The drawing under review shows one solid part. Ordinate dimensions are in mm from its lowest x, y, z. A direction names the side the tool comes from. Coordinates: 2 decimals unless noted, no trailing zeros. Write each loop counter-clockwise with the first axis right and the second up, starting at its lowest first coordinate (ties: lowest second). Pieces come first, ordered by that corner, then holes.
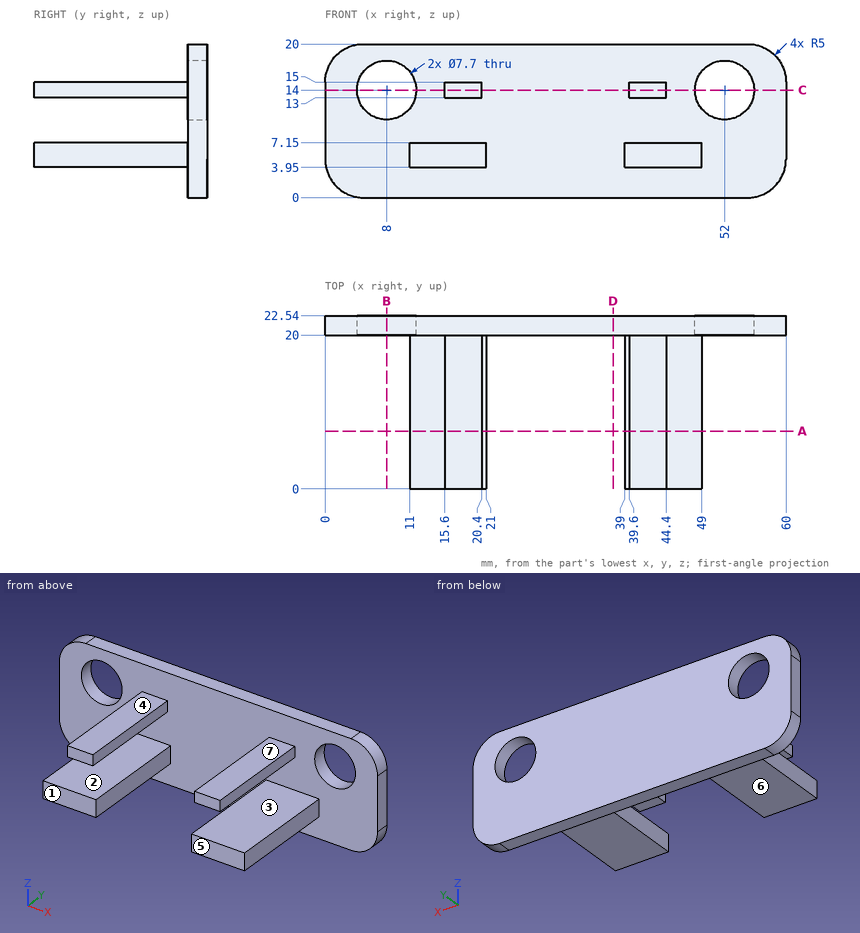
Q1. For probe 1 along X at (y, z) = (21.2, 14); probe 2 along X at (y, z) = (2, 4); probe 3 along Y at (x, z) = (16.5, 17), list the stretches that pass through material, from the lowest coordinate up.
Ans:
probe 1: x = 0 to 4.15, 11.85 to 48.15, 55.85 to 60
probe 2: x = 11 to 21, 39 to 49
probe 3: y = 20 to 22.54
Q2. Clearance check with flat-ended pins moving along their axes: pin 1 Ø9 at (x, z) = (8, 14) entering from +Y; pin 2 Ø1 at (y, z) = (6.5, 6) entering from -X; pin 3 Ø1 at (y, z) = (10.5, 14) entering from +X; pin 4 Ø5 at (x, y) = (16.5, 11) entering from -Z. State where each tip first meets the part, or that it passes through.
Ans:
pin 1: stops at y = 22.54
pin 2: stops at x = 11
pin 3: stops at x = 44.4
pin 4: stops at z = 3.95
Q3. Draft analysis for pull direction Z (two halves, no side actions). For the marked faces 1, 2, 3 and 4, state which applies: +Z half, -Z half, draft (parallel to the pull), parting line (faces both ways), or undercut.
Ans:
face 1: draft
face 2: undercut
face 3: undercut
face 4: +Z half
Q4. Add section A-A (y = 7.5). State the section outline as (x, z) points.
Ans:
outline: (11, 3.95) - (21, 3.95) - (21, 7.15) - (11, 7.15) - close; (15.6, 13) - (20.4, 13) - (20.4, 15) - (15.6, 15) - close; (39, 3.95) - (49, 3.95) - (49, 7.15) - (39, 7.15) - close; (39.6, 13) - (44.4, 13) - (44.4, 15) - (39.6, 15) - close
Q5. Tool access review of the marked faces 5, 6 and 7: name each direction out of +Z, -Z, +X, -X, +Y, -Y from which nothing blocks a thin tool from reaching the whole face with its end or side.
Ans:
face 5: +Z, -Z, +X, -X, -Y
face 6: -Z, +X, -X, -Y
face 7: +Z, +X, -X, -Y
Q6. Add section B-B (x = 8). State the section outline as (y, z) points, then the cut area to 3 significant figures.
Ans:
outline: (20, 0) - (22.54, 0) - (22.54, 10.15) - (20, 10.15) - close; (20, 17.85) - (22.54, 17.85) - (22.54, 20) - (20, 20) - close
area: 31.2 mm2
Q7. Add section C-C (z = 14). State the section outline as (x, y) points, then the cut area to 3 significant figures.
Ans:
outline: (0, 20) - (4.15, 20) - (4.15, 22.54) - (0, 22.54) - close; (11.85, 20) - (15.6, 20) - (15.6, 0) - (20.4, 0) - (20.4, 20) - (39.6, 20) - (39.6, 0) - (44.4, 0) - (44.4, 20) - (48.15, 20) - (48.15, 22.54) - (11.85, 22.54) - close; (55.85, 20) - (60, 20) - (60, 22.54) - (55.85, 22.54) - close
area: 305 mm2
Q8. Add section D-D (x = 37.5). State the section outline as (y, z) points, then the cut area to 3 significant figures.
Ans:
outline: (20, 0) - (22.54, 0) - (22.54, 20) - (20, 20) - close
area: 50.8 mm2
